Geometry check sheet. Reference: the model listing, model coordinates, mm. Round coordinates to 2 decimals unless told otherwise and drop trailing zeros. Write each loop counter-clockwise with the first axis right and the second up, starting at its lowest first coordinate (ties: lowest second). Pieces come first, ordered by that corner, then holes. Notation, with made-up numbers: (75.25, 63) - (114.25, 63) arc R24 ccw to (114.25, 101) - close; hole circle Ø10 at (-26, 56.5). An arc over 180 degrees is marked (long way). Return JSON: item names as keys, results as strings.
```python
from build123d import *

# Parameters (mm, degrees)
SKETCH1_R           = 78.359
SKETCH1_R_2         = 76.1746
BOSS_EXTRUDE1_DEPTH = 977.9
SKETCH2_R           = 1.0922
CUT_EXTRUDE1_DEPTH  = 985.158867136
CIRPATTERN1_COUNT   = 4
CIRPATTERN2_COUNT   = 4


with BuildPart() as part:
    # Sketch1 → Boss-Extrude1 (new body)
    with BuildSketch(Plane(origin=(0, 0, 0), x_dir=(1, 0, 0), z_dir=(0, 1, 0))):
        with Locations(Location((0, 0, 0), (0, 0, 270))):
            Circle(SKETCH1_R)
        with Locations(Location((0, 0, 0), (0, 0, 270))):
            Circle(SKETCH1_R_2, mode=Mode.SUBTRACT)
    extrude(amount=BOSS_EXTRUDE1_DEPTH)

    # Sketch2 → Cut-Extrude1 (cut, through all)
    with BuildSketch(Plane(origin=(0, 0, 0), x_dir=(0, 0, -1), z_dir=(1, 0, 0))):
        with Locations((0, 939.8)):
            Circle(SKETCH2_R)
    cut_extrude1 = extrude(amount=-CUT_EXTRUDE1_DEPTH, mode=Mode.SUBTRACT)

    # CirPattern1: Cut-Extrude1 ×4 about axis
    cirpattern1_axis = Axis((0, 977.9, 0), (0, 1, 0))
    for i in range(1, CIRPATTERN1_COUNT):
        add(cut_extrude1.rotate(cirpattern1_axis, i * 360 / CIRPATTERN1_COUNT), mode=Mode.SUBTRACT)

    # Sketch4 → 1_2 Clearance Hole1 (revolve, cut)
    with BuildSketch(Plane.ZX.offset(111.125)):
        Polygon((0, 0), (0, 92.834507437), (6.54812, 88.9), (6.54812, 0), align=None)
    revolve(axis=Axis((-6.35, 111.125, 0), (1, 0, 0)), mode=Mode.SUBTRACT)

    # Sketch6 → 4.0 _4_ Diameter Hole1 (revolve, cut)
    with BuildSketch(Plane(origin=(0, 101.6, 0), x_dir=(0.7071067811865488, 0, -0.7071067811865464), z_dir=(0, 1, 0))):
        Polygon((0, 0), (0, 90.101721238), (2, 88.9), (2, 0), align=None)
    f_4_0_4_diameter_hole1 = revolve(axis=Axis((4.490128061, 101.6, 4.490128061), (-0.7071067811865464, 0, -0.7071067811865487)), mode=Mode.SUBTRACT)

    # CirPattern2: 4.0 _4_ Diameter Hole1 ×4 about axis
    cirpattern2_axis = Axis((0, 0, 0), (0, 1, 0))
    for i in range(1, CIRPATTERN2_COUNT):
        add(f_4_0_4_diameter_hole1.rotate(cirpattern2_axis, i * 360 / CIRPATTERN2_COUNT), mode=Mode.SUBTRACT)


solid = part.part
```
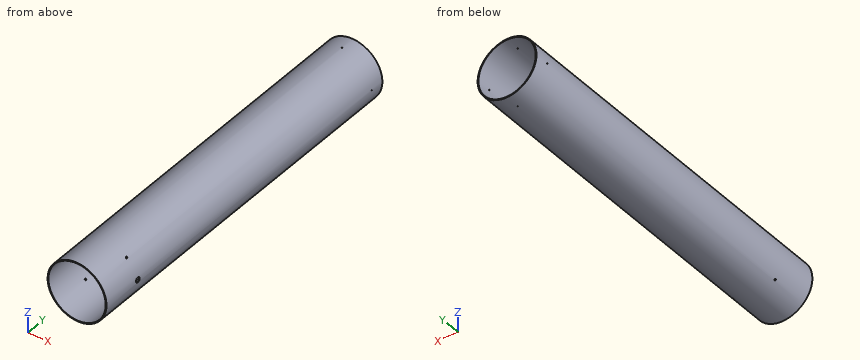
(1) Material ranges on line 1 along Y through (x, z) = (77.85, 0); line 2 along X through (y, z) = (249, 0); line 3 along Z through (x, y) = (-2.5, 289), recorded low to high. Write a range as [from, to].
Response values:
{"line 1": "y = [0, 104.58], [117.67, 938.71], [940.89, 977.9]", "line 2": "x = [-78.36, -76.17], [76.17, 78.36]", "line 3": "z = [-78.32, -76.13], [76.13, 78.32]"}
(2) Section check B-B, the plane y = 786.5. Enter the section's corners in (x, z), plus the area to 3 significant figures.
Response values:
{"outline": "circle Ø156.72 at (0, 0); hole circle Ø152.35 at (0, 0)", "area": "1,060 mm^2"}
(3) Gauge pin test, flat ends, axial feed: pin 1 (6 mm diameter, centred on y = 825, z = -51, fed in from +X); pin 2 (1 mm diameter, centred on x = 51, y = 874.5, fed in from +Z); pin 3 (8 mm diameter, centred on x = -30.5, y = 495.5, fed in from +Z); pin 4 (2.5 mm diameter, centred on x = 0, y = 939.8, fed in from -Z). Record the tip position at first contact, or that the pin passes through.
Response values:
{"pin 1": "stops at x = 61.94", "pin 2": "stops at z = 59.92", "pin 3": "stops at z = 73.74", "pin 4": "stops at z = -78.36"}
